Verification items for the finished model (mm, model axes). A direction names the side the tool comes from. Give positions to 0.01 mm unless a question says otherwise; leave off trailing zeros. Order: outer loops, then holes, each group sorted by start corner. A loop starts at its lowest first (then second) coordinate and runs counter-clockwise, first axis right, second up. Notation, with made-up numbers: M 81.25,87 L 99.25,87 A23 cw 99.25,118 Z; hole C 71,-15 d11. An arc over 180 degrees is marked long. Answer as a JSON object with one key per item and string values.
```python
from build123d import *

# Parameters (mm, degrees)
CUT_EXTRUDE1_DEPTH = 11


with BuildPart() as part:
    # Sketch1 → Revolve1 (revolve)
    with BuildSketch(Plane.XY):
        Polygon((-5, 0), (-5, 20), (-3.5, 20), (-3.5, 15), (3.5, 15), (3.5, 20), (5, 20), (5, 0), align=None)
    revolve(axis=Axis((5, 0, 0), (-1, 0, 0)))

    # Sketch2 → Cut-Extrude1 (cut, through all)
    with BuildSketch(Plane(origin=(5, 0, 0), x_dir=(0, 0, -1), z_dir=(1, 0, 0))):
        with BuildLine():
            Line((1.66945, 1.689108258), (-1.66945, 1.689108258))
            ThreePointArc((-1.66945, 1.689108258), (-0.915252207, -2.191452351), (2.3749, 0))
            ThreePointArc((2.3749, 0), (2.191452351, 0.915252207), (1.66945, 1.689108258))
        make_face()
    extrude(amount=-CUT_EXTRUDE1_DEPTH, mode=Mode.SUBTRACT)


solid = part.part
```
Q1. Material ranges on L1, parallel to Y at x = -2, z = 0; L2, parallel to Z at x = 2.25, y = 0; L3, parallel to Z at x = 2.5, y = -1.5, recorded low to high.
Resolved:
{"L1": "y = -15 to -2.37, 1.69 to 15", "L2": "z = -15 to -2.37, 2.37 to 15", "L3": "z = -14.92 to -1.84, 1.84 to 14.92"}
Q2. Gauge pin test, flat ends, axial feed: pin 1 Ø1.5 at (x, y) = (-4, -3) entering from +Z; pin 2 Ø1 at (x, z) = (1.5, 13.5) entering from -Y; pin 3 Ø4 at (x, y) = (2, 6) entering from -Z. Record the tip position at first contact, or that the pin passes through.
Resolved:
{"pin 1": "stops at z = 19.87", "pin 2": "stops at y = -7.48", "pin 3": "stops at z = -19.45"}
Q3. Section check C-C on z = -10. Record the cut outline in (x, y).
Resolved:
{"outline": "M -5,-17.32 L -3.5,-17.32 L -3.5,-11.18 L 3.5,-11.18 L 3.5,-17.32 L 5,-17.32 L 5,17.32 L 3.5,17.32 L 3.5,11.18 L -3.5,11.18 L -3.5,17.32 L -5,17.32 Z"}
Q4. Section check B-B on x = 2.5. Record the cut outline in (y, z), then the cut area to 3 significant figures.
Resolved:
{"outline": "C 0,0 d30; hole M 1.69,-1.67 L 1.69,1.67 A2.37 ccw long Z", "area": "691 mm²"}
Q5. Release check for a two-part mould opening along X. For faces 4 (the face through (-3.5, 3, -15)), 5 (the face through (4.26, -4.336, 19.524)), 6 (the face through (-5, -4, 0)) record: +X half, -X half, draft (parallel to the pull), parting line (faces both ways), or undercut.
Resolved:
{"face 4": "undercut", "face 5": "draft", "face 6": "-X half"}
Q6. Tool access check on faces 1 (the face through (0, 1.689, 0)), 2 (the face through (3.5, -3, -15)), 3 (the face through (5, 4, 0)). Record the directions out of +Z, -Z, +X, -X, +Y, -Y that give a thin tool (end or side, any length) a straight path to the whole face; none if there is none.
Resolved:
{"face 1": "+X, -X", "face 2": "none", "face 3": "+Z, -Z, +X, +Y, -Y"}
Q7. Section check D-D on y = 4. Record the cut outline in (x, z), then the cut area to 3 significant figures.
Resolved:
{"outline": "M -5,-19.6 L -3.5,-19.6 L -3.5,-14.46 L 3.5,-14.46 L 3.5,-19.6 L 5,-19.6 L 5,19.6 L 3.5,19.6 L 3.5,14.46 L -3.5,14.46 L -3.5,19.6 L -5,19.6 Z", "area": "320 mm²"}
Q8. Section check A-A on z = 0. Record the cut outline in (x, y), then the cut area to 3 significant figures.
Resolved:
{"outline": "M -5,-20 L -3.5,-20 L -3.5,-15 L 3.5,-15 L 3.5,-20 L 5,-20 L 5,-2.37 L -5,-2.37 Z; M -5,1.69 L 5,1.69 L 5,20 L 3.5,20 L 3.5,15 L -3.5,15 L -3.5,20 L -5,20 Z", "area": "289 mm²"}
